```python
from build123d import *

# Parameters (mm, degrees)
SUPPORT_BALISE_W                           = 20
SUPPORT_BALISE_H                           = 350
SUPPORT_BALISE_BOSSAGE_DEPTH               = 80
ESQUISSE3_W                                = 80
ESQUISSE3_H                                = 80
SUPPORT_CHEVAL_ENLEVEMENT_DE_MATIERE_DEPTH = 10
ESQUISSE8_W                                = 10
ESQUISSE8_H                                = 70
SUPPORT_CHEVAL_DEPTH                       = 80
VIS_REACH                                  = 376.466
SERRAGE_VIS_R                              = 2.5
VIS_DIRECTION_2_DEPTH                      = 375.466286867
ENL_V_MAT_EXTRU_5_DEPTH                    = 20
POUR_IMPRESSION_R                          = 15
FIXATION_POUR_ASSEMBLAGE_R                 = 2
VIS_POUR_ASSEMBLAGE_DEPTH                  = 20
ESQUISSE13_R                               = 2
ENL_V_MAT_EXTRU_10_DEPTH                   = 463


with BuildPart() as part:
    # Support Balise → Support balise bossage (new body)
    with BuildSketch(Plane.XY):
        with Locations((10, 175)):
            Rectangle(SUPPORT_BALISE_W, SUPPORT_BALISE_H)
    extrude(amount=SUPPORT_BALISE_BOSSAGE_DEPTH)

    # Esquisse3 → Support Cheval enlevement de matiere (add)
    with BuildSketch(Plane(origin=(0, 350, 0), x_dir=(1, 0, 0), z_dir=(0, 1, 0))):
        with Locations((-20, -40)):
            Rectangle(ESQUISSE3_W, ESQUISSE3_H)
    extrude(amount=SUPPORT_CHEVAL_ENLEVEMENT_DE_MATIERE_DEPTH)

    # Esquisse8 → Support Cheval (cut)
    with BuildSketch(Plane.XY.offset(80)):
        with Locations((10, 35)):
            Rectangle(ESQUISSE8_W, ESQUISSE8_H)
    extrude(amount=-SUPPORT_CHEVAL_DEPTH, mode=Mode.SUBTRACT)

    # Vis: up to this face of the body (flat: up to its plane)
    vis_end = Plane(part.part.faces().sort_by_distance((0, 175, 40))[0])
    # Serrage vis → Vis (cut, up to the picked face)
    with BuildSketch(Plane(origin=(5, 0, 0), x_dir=(0, 0, -1), z_dir=(1, 0, 0)), mode=Mode.PRIVATE) as vis_sk1:
        with Locations((-70, 11.284552026)):
            Circle(SERRAGE_VIS_R)
    vis_tool1 = split(extrude(vis_sk1.sketch, amount=-VIS_REACH, mode=Mode.PRIVATE), bisect_by=vis_end, keep=Keep.BOTH, mode=Mode.PRIVATE)
    # Serrage vis → Vis (cut, up to the picked face)
    with BuildSketch(Plane(origin=(5, 0, 0), x_dir=(0, 0, -1), z_dir=(1, 0, 0)), mode=Mode.PRIVATE) as vis_sk2:
        with Locations((-70, 53.057184379)):
            Circle(SERRAGE_VIS_R)
    vis_tool2 = split(extrude(vis_sk2.sketch, amount=-VIS_REACH, mode=Mode.PRIVATE), bisect_by=vis_end, keep=Keep.BOTH, mode=Mode.PRIVATE)
    # Serrage vis → Vis (cut, up to the picked face)
    with BuildSketch(Plane(origin=(5, 0, 0), x_dir=(0, 0, -1), z_dir=(1, 0, 0)), mode=Mode.PRIVATE) as vis_sk3:
        with Locations((-10, 53.057184379)):
            Circle(SERRAGE_VIS_R)
    vis_tool3 = split(extrude(vis_sk3.sketch, amount=-VIS_REACH, mode=Mode.PRIVATE), bisect_by=vis_end, keep=Keep.BOTH, mode=Mode.PRIVATE)
    # Serrage vis → Vis (cut, up to the picked face)
    with BuildSketch(Plane(origin=(5, 0, 0), x_dir=(0, 0, -1), z_dir=(1, 0, 0)), mode=Mode.PRIVATE) as vis_sk4:
        with Locations((-10, 11.284552026)):
            Circle(SERRAGE_VIS_R)
    vis_tool4 = split(extrude(vis_sk4.sketch, amount=-VIS_REACH, mode=Mode.PRIVATE), bisect_by=vis_end, keep=Keep.BOTH, mode=Mode.PRIVATE)
    # Serrage vis → Vis (cut, up to the picked face)
    with BuildSketch(Plane(origin=(5, 0, 0), x_dir=(0, 0, -1), z_dir=(1, 0, 0)), mode=Mode.PRIVATE) as vis_sk5:
        with Locations((-40, 32.170868202)):
            Circle(SERRAGE_VIS_R)
    vis_tool5 = split(extrude(vis_sk5.sketch, amount=-VIS_REACH, mode=Mode.PRIVATE), bisect_by=vis_end, keep=Keep.BOTH, mode=Mode.PRIVATE)
    add(vis_tool1.solids().sort_by(Axis((5, 11.284552, 70), (-1, 0, 0)))[0], mode=Mode.SUBTRACT)
    add(vis_tool2.solids().sort_by(Axis((5, 53.057184, 70), (-1, 0, 0)))[0], mode=Mode.SUBTRACT)
    add(vis_tool3.solids().sort_by(Axis((5, 53.057184, 10), (-1, 0, 0)))[0], mode=Mode.SUBTRACT)
    add(vis_tool4.solids().sort_by(Axis((5, 11.284552, 10), (-1, 0, 0)))[0], mode=Mode.SUBTRACT)
    add(vis_tool5.solids().sort_by(Axis((5, 32.170868, 40), (-1, 0, 0)))[0], mode=Mode.SUBTRACT)

    # Serrage vis → Vis direction 2 (cut)
    with BuildSketch(Plane(origin=(5, 0, 0), x_dir=(0, 0, -1), z_dir=(1, 0, 0))):
        with Locations((-70, 11.284552026)):
            Circle(SERRAGE_VIS_R)
        with Locations((-70, 53.057184379)):
            Circle(SERRAGE_VIS_R)
        with Locations((-10, 53.057184379)):
            Circle(SERRAGE_VIS_R)
        with Locations((-10, 11.284552026)):
            Circle(SERRAGE_VIS_R)
        with Locations((-40, 32.170868202)):
            Circle(SERRAGE_VIS_R)
    extrude(amount=VIS_DIRECTION_2_DEPTH, mode=Mode.SUBTRACT)

    # Design → Enlèv. mat.-Extru.5 (cut)
    with BuildSketch(Plane(origin=(20, 0, 0), x_dir=(0, 0, -1), z_dir=(1, 0, 0))):
        Polygon((-55, 315), (-80, 360), (-80, 92.406088827), (-55, 137.406088827), align=None)
        Polygon((0, 92.406088827), (0, 360), (-25, 315), (-25, 137.406088827), align=None)
    extrude(amount=-ENL_V_MAT_EXTRU_5_DEPTH, mode=Mode.SUBTRACT)

    # Pour Impression
    # the kernel refuses this fillet: 15 mm, written as the material it adds along each edge
    with BuildSketch(Plane(origin=(0, 392.780897855, -18.211609919), x_dir=(1, 0, 0), z_dir=(0, -0.8741572761215375, 0.48564293117863266))) as pour_impression_piece_1_section:
        with BuildLine():
            CenterArc((POUR_IMPRESSION_R, -POUR_IMPRESSION_R), POUR_IMPRESSION_R, 90, 90)
            Line((0, -POUR_IMPRESSION_R), (0, 0))
            Line((0, 0), (POUR_IMPRESSION_R, 0))
        make_face()
    pour_impression_piece_1 = extrude(amount=86.439589046, mode=Mode.PRIVATE)
    pour_impression_piece_1 = split(pour_impression_piece_1, bisect_by=Plane(origin=(4.741525676, 350, 2.029382941), z_dir=(0, 1, 0)), keep=Keep.TOP, mode=Mode.PRIVATE)
    pour_impression_piece_1 = split(pour_impression_piece_1, bisect_by=Plane(origin=(4.741525676, 353.652889294, 0), z_dir=(0, 0, 1)), keep=Keep.TOP, mode=Mode.PRIVATE)
    add(pour_impression_piece_1)
    with BuildSketch(Plane(origin=(0, 317.219102145, 56.232834525), x_dir=(1, 0, 0), z_dir=(0, 0.8741572761215377, 0.4856429311786322))) as pour_impression_piece_2_section:
        with BuildLine():
            CenterArc((POUR_IMPRESSION_R, -POUR_IMPRESSION_R), POUR_IMPRESSION_R, 90, 90)
            Line((0, -POUR_IMPRESSION_R), (0, 0))
            Line((0, 0), (POUR_IMPRESSION_R, 0))
        make_face()
    pour_impression_piece_2 = extrude(amount=86.439589046, mode=Mode.PRIVATE)
    pour_impression_piece_2 = split(pour_impression_piece_2, bisect_by=Plane(origin=(4.741525676, 350, 77.970617059), z_dir=(0, 1, 0)), keep=Keep.TOP, mode=Mode.PRIVATE)
    pour_impression_piece_2 = split(pour_impression_piece_2, bisect_by=Plane(origin=(4.741525676, 353.652889294, 80), z_dir=(0, 0, -1)), keep=Keep.TOP, mode=Mode.PRIVATE)
    add(pour_impression_piece_2)

    # Fixation pour assemblage → Vis pour Assemblage (cut)
    with BuildSketch(Plane(origin=(20, 0, 0), x_dir=(0, 0, -1), z_dir=(1, 0, 0))):
        with Locations((-47.5, 195)):
            Circle(FIXATION_POUR_ASSEMBLAGE_R)
        with Locations((-32.5, 195)):
            Circle(FIXATION_POUR_ASSEMBLAGE_R)
        with Locations((-32.5, 175)):
            Circle(FIXATION_POUR_ASSEMBLAGE_R)
        with Locations((-47.5, 175)):
            Circle(FIXATION_POUR_ASSEMBLAGE_R)
    extrude(amount=-VIS_POUR_ASSEMBLAGE_DEPTH, mode=Mode.SUBTRACT)

    # Esquisse13 → Enlèv. mat.-Extru.10 (cut)
    # profile 1 of 2: a face of its own
    with BuildSketch(Plane(origin=(20, 0, 0), x_dir=(0, 0, -1), z_dir=(1, 0, 0))):
        Polygon((-174.897376457, 185), (-55, 185), (-55, 315), (-80, 360), (0, 360), (-25, 315), (-25, 185), (122.454281653, 185), (122.454281653, 440.420380727), (-174.897376457, 440.420380727), align=None)
    # profile 2 of 2: a face of its own
    with BuildSketch(Plane(origin=(20, 0, 0), x_dir=(0, 0, -1), z_dir=(1, 0, 0))):
        Polygon((-55, 315), (-55, 185), (-25, 185), (-25, 315), (0, 360), (-80, 360), align=None)
        with Locations((-47.5, 195)):
            Circle(ESQUISSE13_R, mode=Mode.SUBTRACT)
        with Locations((-32.5, 195)):
            Circle(ESQUISSE13_R, mode=Mode.SUBTRACT)
    extrude(amount=-ENL_V_MAT_EXTRU_10_DEPTH, mode=Mode.SUBTRACT)


solid = part.part
```
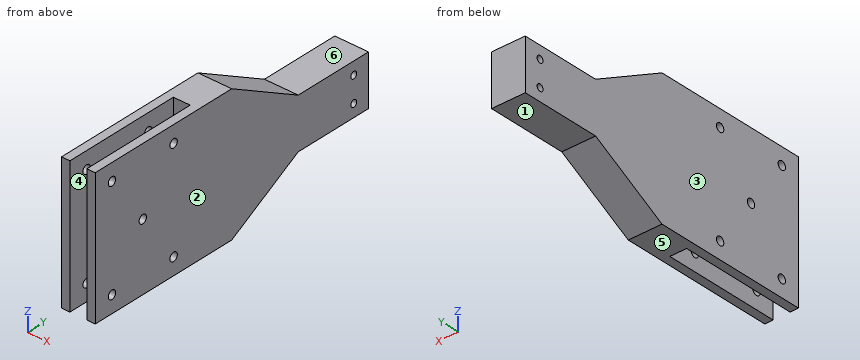
For this review, take the finished solid that the model builds, in its own axes (mm). Face numbers are marked on the shaded views. A direction names the side the tool comes from. Give positions to 0.01 mm unless a question says otherwise; leave off trailing zeros. Write each loop counter-clockwise with the first axis right and the second up, starting at its lowest first coordinate (ties: lowest second). Pieces come first, ordered by that corner, then holes. Notation, with made-up numbers: M 74,75 L 131,75 A4 ccw 131,79 Z; hole C 7.25,-5 d4. An arc over 180 degrees is marked long. Answer as a JSON object with one key per item and string values. Group by question number.
Item 1: Draft analysis for pull direction X (two halves, no side actions). For the marked faces 1, 2, 3 and 4, state which applies: +X half, -X half, draft (parallel to the pull), parting line (faces both ways), or undercut.
Item 2: For probe 1 along Z at (x, y) = (8.75, 175); probe 2 along Y at (x, z) = (2, 10); probe 3 along Y at (x, z) = (9.5, 32.5), list the stretches that pass through material, from the lowest coordinate up. Write a range as [from, to].
Item 3: Consider section A-A on y = 175. Write out the cut boundary in (x, z), plus the area to 3 significant figures.
Item 4: Tool access review of the marked faces 5 and 6: name each direction out of +Z, -Z, +X, -X, +Y, -Y from which nothing blocks a thin tool from reaching the whole face with its end or side.
Item 5: Consider section B-B on z = 32.5. Write out the cut boundary in (x, y), plus the area to 3 significant figures.
Item 6: For pin 1 Ø10 at (x, y) = (12.5, 165) entering from -Z; pin 2 Ø3 at (y, z) = (79, 31) entering from -X; pin 3 Ø1.5 at (x, z) = (12, 25) entering from -Y; pin 4 Ø2 at (x, y) = (5.5, 134) entering from -Z, all flat-tipped, find the tip position at first contact; note any pin that passes through.
Item 7: Consider section D-D on z = 10. Write out the cut boundary in (x, y), plus the area to 3 significant figures.
Item 8: Consider section C-C on x = 10.75. Write out the cut boundary in (y, z).
Check result:
{
 "1": {"face 1": "draft", "face 2": "+X half", "face 3": "-X half", "face 4": "undercut"},
 "2": {"probe 1": "z = [25, 30.5], [34.5, 45.5], [49.5, 55]", "probe 2": "y = [0, 8.78], [13.78, 50.56], [55.56, 110.41]", "probe 3": "y = [70, 173], [177, 185]"},
 "3": {"outline": "M 0,25 L 20,25 L 20,30.5 L 0,30.5 Z; M 0,34.5 L 20,34.5 L 20,45.5 L 0,45.5 Z; M 0,49.5 L 20,49.5 L 20,55 L 0,55 Z", "area": "440 mm^2"},
 "4": {"face 5": "-Z, +X, -X, +Y, -Y", "face 6": "+Z, +X, -X, +Y"},
 "5": {"outline": "M 0,0 L 5,0 L 5,70 L 15,70 L 15,0 L 20,0 L 20,173 L 0,173 Z; M 0,177 L 20,177 L 20,185 L 0,185 Z", "area": "2,920 mm^2"},
 "6": {"pin 1": "stops at z = 25", "pin 2": "stops at x = 0", "pin 3": "stops at y = 70", "pin 4": "stops at z = 22.55"},
 "7": {"outline": "M 0,0 L 5,0 L 5,8.78 L 0,8.78 Z; M 0,13.78 L 5,13.78 L 5,50.56 L 0,50.56 Z; M 0,55.56 L 5,55.56 L 5,70 L 15,70 L 15,55.56 L 20,55.56 L 20,110.41 L 0,110.41 Z; M 15,0 L 20,0 L 20,8.78 L 15,8.78 Z; M 15,13.78 L 20,13.78 L 20,50.56 L 15,50.56 Z", "area": "1,410 mm^2"},
 "8": {"outline": "M 70,0 L 92.41,0 L 137.41,25 L 185,25 L 185,55 L 137.41,55 L 92.41,80 L 70,80 Z; hole C 175,32.5 d4; hole C 175,47.5 d4"}
}
